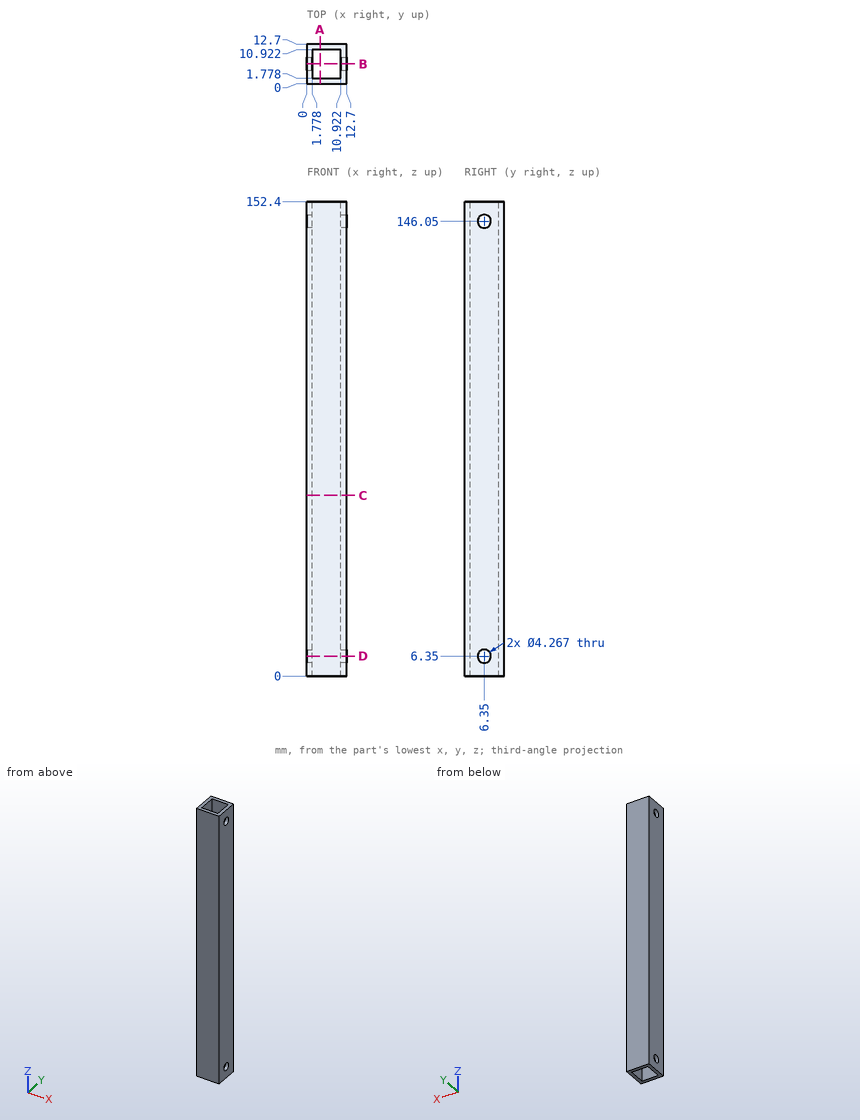
Check sheet for the drawn part. Datum: minimum x, y, z corner. Units: mm. Give positions to 0.01 mm unless a question says otherwise; leave off trailing zeros. Write each loop counter-clockwise with the first axis right and the second up, starting at its lowest first coordinate (ties: lowest second). Pieces come first, ordered by that corner, then holes. Notation, with made-up numbers: (-8.5, -20) -> (45.5, -20) arc R16 ccw to (45.5, 8) -> close; hole circle Ø8 at (11.25, 21). An arc over 180 degrees is marked (long way). Use one line per item in the form item = value. Start each with the question number.
1. Section check B-B (y = 6.35). Record the cut outline in (x, z).
2. Go/stop test with a flat-tipped pin: P1, Ø7, axis at y = 6.35, z = 6.35, coming from the +X side. Record where the tip stops, or that it passes through.
3. Section check D-D (z = 6.35). Record the cut outline in (x, y).
4. Thickness scan on line 1 along Y through (x, z) = (2.25, 120.5); line 2 along Y through (x, z) = (11.95, 6.35). Record the ranges inside material, lowest first. Write a range as from..to.
5. Section check C-C (z = 58). Record the cut outline in (x, y).
6. Section check A-A (x = 4.25). Record the cut outline in (y, z), and give its area (3 significant figures).
Conclusion:
q1.outline = (0, 0) -> (1.78, 0) -> (1.78, 4.22) -> (0, 4.22) -> close; (0, 8.48) -> (1.78, 8.48) -> (1.78, 143.92) -> (0, 143.92) -> close; (0, 148.18) -> (1.78, 148.18) -> (1.78, 152.4) -> (0, 152.4) -> close; (10.92, 0) -> (12.7, 0) -> (12.7, 4.22) -> (10.92, 4.22) -> close; (10.92, 8.48) -> (12.7, 8.48) -> (12.7, 143.92) -> (10.92, 143.92) -> close; (10.92, 148.18) -> (12.7, 148.18) -> (12.7, 152.4) -> (10.92, 152.4) -> close
q2.P1 = 12.7
q3.outline = (0, 0) -> (12.7, 0) -> (12.7, 4.22) -> (10.92, 4.22) -> (10.92, 1.78) -> (1.78, 1.78) -> (1.78, 4.22) -> (0, 4.22) -> close; (0, 8.48) -> (1.78, 8.48) -> (1.78, 10.92) -> (10.92, 10.92) -> (10.92, 8.48) -> (12.7, 8.48) -> (12.7, 12.7) -> (0, 12.7) -> close
q4.line_1 = 0..1.78, 10.92..12.7
q4.line_2 = 0..4.22, 8.48..12.7
q5.outline = (0, 0) -> (12.7, 0) -> (12.7, 12.7) -> (0, 12.7) -> close; hole (1.78, 1.78) -> (10.92, 1.78) -> (10.92, 10.92) -> (1.78, 10.92) -> close
q6.outline = (0, 0) -> (1.78, 0) -> (1.78, 152.4) -> (0, 152.4) -> close; (10.92, 0) -> (12.7, 0) -> (12.7, 152.4) -> (10.92, 152.4) -> close
q6.area = 542 mm²
